```python
from build123d import *

# Parameters (mm, degrees)
SKETCH1_W                      = 38.1
SKETCH1_H                      = 120
BOSS_EXTRUDE1_DEPTH            = 38.1
SKETCH2_W                      = 34.925
SKETCH2_H                      = 34.925
CUT_EXTRUDE1_DEPTH             = 130.767142413
F_4_2_4_2_DIAMETER_HOLE1_D     = 4.2
F_6_0_6_DIAMETER_HOLE1_D       = 6
F_4_2_4_2_DIAMETER_HOLE2_D     = 4.2
F_4_2_4_2_DIAMETER_HOLE2_DEPTH = 38.1
F_6_0_6_DIAMETER_HOLE2_D       = 6
F_6_0_6_DIAMETER_HOLE2_DEPTH   = 38.1
F_6_0_6_DIAMETER_HOLE3_D       = 6
F_6_0_6_DIAMETER_HOLE3_DEPTH   = 38.1
F_4_2_4_2_DIAMETER_HOLE3_D     = 4.2
SKETCH15_R                     = 2.1
SKETCH15_R_2                   = 3
BOSS_EXTRUDE2_DEPTH            = 3.175
BOSS_EXTRUDE3_START            = -3.175
SKETCH16_R                     = 2.1
BOSS_EXTRUDE3_DEPTH            = 3.175
SKETCH18_W                     = 3.175
SKETCH18_H                     = 3.175
CUT_EXTRUDE2_DEPTH             = 130.767142413
CUT_EXTRUDE3_START             = -3.175
CUT_EXTRUDE3_OUTLINE_R         = 2.1
CUT_EXTRUDE3_DEPTH             = 3.175
BOSS_EXTRUDE4_START            = -3.175
BOSS_EXTRUDE4_OUTLINE_R        = 3
BOSS_EXTRUDE4_DEPTH            = 3.175
SKETCH19_R                     = 3
CUT_EXTRUDE4_DEPTH             = 121.228267267


# Read off the part's stored shape, not the designer's step: Cut-Extrude3, Boss-Extrude4
with BuildPart() as part:
    # Sketch1 → Boss-Extrude1 (new body)
    with BuildSketch(Plane.XZ.offset(34.925)):
        with Locations((15.875, -55)):
            Rectangle(SKETCH1_W, SKETCH1_H)
    extrude(amount=-BOSS_EXTRUDE1_DEPTH)

    # Sketch2 → Cut-Extrude1 (cut, through all)
    with BuildSketch(Plane(origin=(0, 0, -115), x_dir=(-1, 0, 0), z_dir=(0, 0, -1))):
        with Locations((-17.4625, -17.4625)):
            Rectangle(SKETCH2_W, SKETCH2_H)
    extrude(amount=-CUT_EXTRUDE1_DEPTH, mode=Mode.SUBTRACT)

    # Ø4.2 (4.2) Diameter Hole1 (through all)
    with Locations(Plane(origin=(0, 0, 0), x_dir=(-1, 0, 0), z_dir=(0, -1, 0))):
        with Locations((-5, 35.97), (-5, 91.03)):
            Hole(F_4_2_4_2_DIAMETER_HOLE1_D / 2)

    # Ø6.0 (6) Diameter Hole1 (through all)
    with Locations(Plane(origin=(0, 0, 0), x_dir=(-1, 0, 0), z_dir=(0, -1, 0))):
        with Locations((-22.225, 106.5), (-22.225, 46.5)):
            Hole(F_6_0_6_DIAMETER_HOLE1_D / 2)

    # Ø4.2 (4.2) Diameter Hole2
    with Locations(Plane(origin=(0, 3.175, 0), x_dir=(1, 0, 0), z_dir=(0, 1, 0))):
        with Locations((22.225, 33.5), (22.225, 93.5), (29.296067812, 100.571067812), (29.296067812, 26.428932188)):
            Hole(F_4_2_4_2_DIAMETER_HOLE2_D / 2, depth=F_4_2_4_2_DIAMETER_HOLE2_DEPTH)

    # Ø6.0 (6) Diameter Hole2
    with Locations(Plane(origin=(0, 3.175, 0), x_dir=(1, 0, 0), z_dir=(0, 1, 0))):
        with Locations((24.925, 6)):
            Hole(F_6_0_6_DIAMETER_HOLE2_D / 2, depth=F_6_0_6_DIAMETER_HOLE2_DEPTH)

    # Ø6.0 (6) Diameter Hole3
    with Locations(Plane.ZY.offset(3.175)):
        with Locations((-6, -24.925), (-106.5, -22.225), (-46.5, -22.225)):
            Hole(F_6_0_6_DIAMETER_HOLE3_D / 2, depth=F_6_0_6_DIAMETER_HOLE3_DEPTH)

    # Ø4.2 (4.2) Diameter Hole3 (through all)
    with Locations(Plane.ZY.offset(3.175)):
        with Locations((-93.5, -22.225), (-33.5, -22.225), (-35.97, -5), (-91.03, -5), (-100.571067812, -29.296067812), (-26.428932188, -29.296067812)):
            Hole(F_4_2_4_2_DIAMETER_HOLE3_D / 2)

    # Sketch15 → Boss-Extrude2 (add)
    with BuildSketch(Plane(origin=(0, 3.175, 0), x_dir=(1, 0, 0), z_dir=(0, 1, 0))):
        with Locations((29.296067812, 26.428932188)):
            Circle(SKETCH15_R)
        with Locations((29.296067812, 100.571067812)):
            Circle(SKETCH15_R)
        with Locations((22.225, 106.5)):
            Circle(SKETCH15_R_2)
        with Locations((22.225, 46.5)):
            Circle(SKETCH15_R_2)
        with Locations((5, 35.97)):
            Circle(SKETCH15_R)
        with Locations((5, 91.03)):
            Circle(SKETCH15_R)
    extrude(amount=-BOSS_EXTRUDE2_DEPTH)

    # Sketch16 → Boss-Extrude3 (add)
    with BuildSketch(Plane.ZY.offset(3.175).offset(BOSS_EXTRUDE3_START)):
        with Locations((-100.571067812, -29.296067812)):
            Circle(SKETCH16_R)
        with Locations((-26.428932188, -29.296067812)):
            Circle(SKETCH16_R)
        with Locations((-35.97, -5)):
            Circle(SKETCH16_R)
        with Locations((-91.03, -5)):
            Circle(SKETCH16_R)
    extrude(amount=BOSS_EXTRUDE3_DEPTH)

    # Sketch18 → Cut-Extrude2 (cut, through all)
    with BuildSketch(Plane.XY.offset(5)):
        with Locations((-1.5875, 1.5875)):
            Rectangle(SKETCH18_W, SKETCH18_H)
    extrude(amount=-CUT_EXTRUDE2_DEPTH, mode=Mode.SUBTRACT)


with BuildPart() as body_2:
    # of the pieces the cut leaves, the one that is kept (cut_extrude2_keep)
    add(part.part.solids().sort_by_distance((-3.175, -34.925, -115))[0])

    # Cut-Extrude3 outline → Cut-Extrude3 (cut)
    with BuildSketch(Plane.YZ.offset(CUT_EXTRUDE3_START)):
        with Locations((-5, -91.03)):
            Circle(CUT_EXTRUDE3_OUTLINE_R)
        with Locations((-5, -35.97)):
            Circle(CUT_EXTRUDE3_OUTLINE_R)
        with Locations((-29.296067812, -26.428932188)):
            Circle(CUT_EXTRUDE3_OUTLINE_R)
        with Locations((-29.296067812, -100.571067812)):
            Circle(CUT_EXTRUDE3_OUTLINE_R)
    extrude(amount=CUT_EXTRUDE3_DEPTH, mode=Mode.SUBTRACT)

    # Boss-Extrude4 outline → Boss-Extrude4 (add)
    with BuildSketch(Plane.YZ.offset(BOSS_EXTRUDE4_START)):
        with Locations((-22.225, -46.5)):
            Circle(BOSS_EXTRUDE4_OUTLINE_R)
        with Locations((-22.225, -106.5)):
            Circle(BOSS_EXTRUDE4_OUTLINE_R)
        with Locations((-24.925, -6)):
            Circle(BOSS_EXTRUDE4_OUTLINE_R)
    extrude(amount=BOSS_EXTRUDE4_DEPTH)

    # Sketch19 → Cut-Extrude4 (cut, through all)
    with BuildSketch(Plane.ZY.offset(3.175)):
        with Locations((-93.8, -17.4625)):
            Circle(SKETCH19_R)
        with Locations((-33.8, -17.4625)):
            Circle(SKETCH19_R)
        with Locations((-6, -4.7625)):
            Circle(SKETCH19_R)
        with Locations((-6, -30.1625)):
            Circle(SKETCH19_R)
    extrude(amount=-CUT_EXTRUDE4_DEPTH, mode=Mode.SUBTRACT)


solid = body_2.part
```
Work out the finished part from the listing and answer in its coordinate system (mm). Round coordinates to 2 decimals unless told otherwise and drop trailing zeros. Return JSON: item names as keys, results as strings. Group by question number.
Q1. Find the intervals of material crossed by L1, parallel to Y at x = -1.55, z = -6 (1 decimal); L2, parallel to Z at x = -2.3, y = -5; L3, parallel to Y at x = -0.7, z = -93.8 (1 decimal), in increasing order.
Q2. The part is cut by section A-A on x = -0.6. Count the separate pieces of the cut face and the enclosed holes in it, then the cut area to 3 significant figures.
Q3. The mould has two halves that part along Z. Classify faces 1 (the cylindrical face through (-1.61, -7.424, -4.616)), 2 (the flat face through (-3.175, -18, -54)), 3 (the flat face through (-2, -18, 5)): released by +Z, released by -Z, zero draft, split by the parting line, or undercut.
Solved:
{
 "1": {"L1": "-34.9 to -33.2, -27.2 to -7.8, -1.8 to 0", "L2": "-115 to -93.13, -88.93 to -38.07, -33.87 to -8.99, -3.01 to 5", "L3": "-34.9 to -24.3, -14.5 to 0"},
 "2": {"separate pieces": "1", "enclosed holes": "8", "area": "4,000 mm²"},
 "3": {"face 1": "undercut", "face 2": "zero draft", "face 3": "released by +Z"}
}
